Check sheet for the modelled part. Datum: model origin and axes. Units: mm. Face numbers are marked on the shaded views. Round coordinates to 2 decimals unless told otherwise and drop trailing zeros. Order: outer loops, then holes, each group sorted by start corner. A loop starts at its lowest first (then second) coordinate and runs counter-clockwise, first axis right, second up.
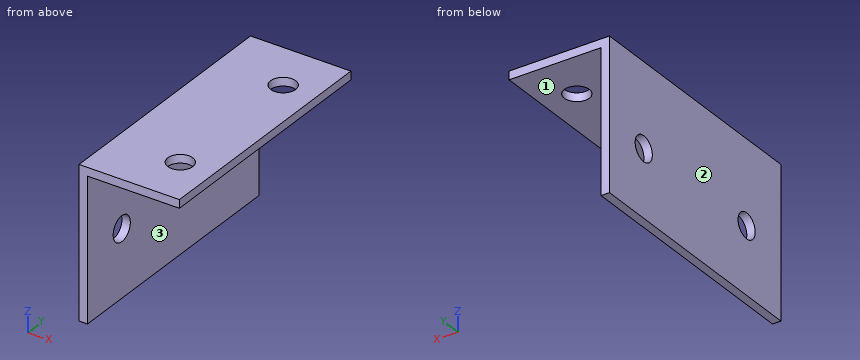
```python
from build123d import *

# Parameters (mm, degrees)
EXTRUDE_2_DEPTH     = 30
SKETCH_5_R          = 1.5
CUT_EXTRUDE_3_DEPTH = 37.510272527
SKETCH_6_R          = 1.5
CUT_EXTRUDE_4_DEPTH = 37.674241642


with BuildPart() as part:
    # 草图4 → 凸台-拉伸2 (new body)
    with BuildSketch(Plane(origin=(0, 0, 0), x_dir=(1, 0, 0), z_dir=(0, 1, 0))):
        Polygon((0, 0), (0, 18), (1, 18), (1, 1), (12, 1), (12, 0), align=None)
    extrude(amount=EXTRUDE_2_DEPTH)

    # 草图5 → 切除-拉伸3 (cut, through all)
    with BuildSketch(Plane(origin=(0, 0, -1), x_dir=(-1, 0, 0), z_dir=(0, 0, -1))):
        with Locations((-8, 6)):
            Circle(SKETCH_5_R)
        with Locations(Location((-8, 24, 0), (0, 0, 180))):
            Circle(SKETCH_5_R)
    extrude(amount=-CUT_EXTRUDE_3_DEPTH, mode=Mode.SUBTRACT)

    # 草图6 → 切除-拉伸4 (cut, through all)
    with BuildSketch(Plane(origin=(1, 0, 0), x_dir=(0, 0, -1), z_dir=(1, 0, 0))):
        with Locations((10, 24)):
            Circle(SKETCH_6_R)
        with Locations(Location((10, 6, 0), (0, 0, 180))):
            Circle(SKETCH_6_R)
    extrude(amount=-CUT_EXTRUDE_4_DEPTH, mode=Mode.SUBTRACT)


solid = part.part
```
Item 1: Sectioned sample at A-A (x = 8). Record the cut outline in (y, z), and give its area (3 significant figures).
Answer:
outline: (0, -1) - (4.5, -1) - (4.5, 0) - (0, 0) - close; (7.5, -1) - (22.5, -1) - (22.5, 0) - (7.5, 0) - close; (25.5, -1) - (30, -1) - (30, 0) - (25.5, 0) - close
area: 24.0 mm2
Item 2: Sectioned sample at D-D (y = 9). Record the cut outline in (x, z).
Answer:
outline: (0, -18) - (1, -18) - (1, -1) - (12, -1) - (12, 0) - (0, 0) - close
Item 3: Sectioned sample at B-B (y = 24). Record the cut outline in (x, z), and give its area (3 significant figures).
Answer:
outline: (0, -18) - (1, -18) - (1, -11.5) - (0, -11.5) - close; (0, -8.5) - (1, -8.5) - (1, -1) - (6.5, -1) - (6.5, 0) - (0, 0) - close; (9.5, -1) - (12, -1) - (12, 0) - (9.5, 0) - close
area: 23.0 mm2
Item 4: Go/stop test with flat-tipped pins: P1, Ø4, axis at x = 6, y = 5.5, coming from the +Z side; P2, Ø6, axis at y = 12.5, z = -7, coming from the +X side; P3, Ø2.5, axis at y = 6, z = -10, coming from the +X side; P4, Ø5, axis at x = 8, y = 24, coming from the -Z side. Record where each tip stops, or that it passes through.
Answer:
P1: stops at z = 0
P2: stops at x = 1
P3: passes through
P4: stops at z = -1
Item 5: Sectioned sample at C-C (z = -10). Record the cut outline in (x, y).
Answer:
outline: (0, 0) - (1, 0) - (1, 4.5) - (0, 4.5) - close; (0, 7.5) - (1, 7.5) - (1, 22.5) - (0, 22.5) - close; (0, 25.5) - (1, 25.5) - (1, 30) - (0, 30) - close
Item 6: Scan lines: line 1 along Y through (x, z) = (0.5, -10); line 2 along Z through (x, y) = (0.4, 6); line 3 along X through (y, z) = (2.5, -14). Record each from-to range of solid material in increasing order.
Answer:
line 1: y = 0 to 4.5, 7.5 to 22.5, 25.5 to 30
line 2: z = -18 to -11.5, -8.5 to 0
line 3: x = 0 to 1
Item 7: Release check for a two-part mould opening along X. For the marked faces 1, 2 and 3 record: released by +X, released by -X, zero draft, split by the parting line, or undercut.
Answer:
face 1: zero draft
face 2: released by -X
face 3: released by +X
